Check sheet for the modelled part. Datum: model origin and axes. Units: mm. A direction names the side the tool comes from. Round coordinates to 2 decimals unless told otherwise and drop trailing zeros. Loops run counter-clockwise (first coordinate to the right, second up) from the corner with the lowest first, then second, coordinate; pieces in that order, holes last. Notation, with made-up numbers: (-1.5, 42.5) - (27.5, 42.5) arc R11 cw to (27.5, 60.5) - close; hole circle Ø7 at (29, 79.25). An arc over 180 degrees is marked (long way). Return JSON: item names as keys, results as strings.
from build123d import *

# Parameters (mm, degrees)
EXTRUDE_START            = -3.462177
EXTRUDE_1_DEPTH          = 40
EXTRUDE_START_2          = 60
EXTRUDE_2_DEPTH          = 60
CUT_EXTRUDE_1_REACH      = 163.234
CUT_EXTRUDE_1_END_RADIUS = 128.062484749
SKETCH_1_R               = 25
CUT_EXTRUDE_2_DEPTH      = 163.48076826
CUT_EXTRUDE_2_DEPTH_BACK = 163.48076826
SKETCH_5_R               = 25
SKETCH_5_R_2             = 15


with BuildPart() as part:
    # 草图2 → 凸台-拉伸1 (new body)
    with BuildSketch(Plane.XY.offset(EXTRUDE_START)):
        with BuildLine():
            Line((-80, 0), (80, 0))
            Line((80, 0), (80, 100))
            ThreePointArc((80, 100), (0, 128.062484749), (-80, 100))
            Line((-80, 100), (-80, 0))
        make_face()
    extrude(amount=-EXTRUDE_1_DEPTH)

    # 草图4 → 凸台-拉伸2 (add)
    with BuildSketch(Plane.XY.offset(-3.46217708).offset(EXTRUDE_START_2)):
        with BuildLine():
            Line((-35, 0), (-35, 123.186849948))
            ThreePointArc((-35, 123.186849948), (0, 128.062484749), (35, 123.186849948))
            Line((35, 123.186849948), (35, 0))
            Line((35, 0), (-35, 0))
        make_face()
    extrude(amount=-EXTRUDE_2_DEPTH)

    # 切除-拉伸1: up to this cylinder (the profile starts inside it)
    cut_extrude_1_end = Plane(origin=(0, 0, 6.537823), z_dir=(0, 0, 1)) * Cylinder(CUT_EXTRUDE_1_END_RADIUS, 583.592969497, mode=Mode.PRIVATE)
    # 草图1 → 切除-拉伸1 (cut, up to the surface)
    with BuildSketch(Plane(origin=(0, 0, 0), x_dir=(1, 0, 0), z_dir=(0, 1, 0)), mode=Mode.PRIVATE) as cut_extrude_1_sk1:
        with Locations(Location((0, -6.53782292, 0), (0, 0, 90))):
            Circle(SKETCH_1_R)
    cut_extrude_1_tool1 = extrude(cut_extrude_1_sk1.sketch, amount=CUT_EXTRUDE_1_REACH, mode=Mode.PRIVATE) & cut_extrude_1_end
    add(cut_extrude_1_tool1.solids().sort_by_distance((0, 0, 6.537823))[0], mode=Mode.SUBTRACT)

    # 草图5 → 切除-拉伸2 (cut, two sides: drawn at the far end of the back side and taken through both)
    with BuildSketch(Plane.XY.offset(-3.46217708).offset(-CUT_EXTRUDE_2_DEPTH_BACK)):
        with Locations((0, 70)):
            Circle(SKETCH_5_R)
        with Locations((-55, 50)):
            Circle(SKETCH_5_R_2)
        with Locations((55, 50)):
            Circle(SKETCH_5_R_2)
    extrude(amount=CUT_EXTRUDE_2_DEPTH + CUT_EXTRUDE_2_DEPTH_BACK, mode=Mode.SUBTRACT)


solid = part.part
Q1. Sectioned sample at A-A (x = -5.5). Enter the section's corners in (y, z), plus the area to 3 significant figures.
Answer key:
{"outline": "(0, -43.46) - (45.61, -43.46) - (45.61, -17.85) - (0, -17.85) - close; (0, 30.93) - (45.61, 30.93) - (45.61, 56.54) - (0, 56.54) - close; (94.39, -43.46) - (127.94, -43.46) - (127.94, -17.85) - (94.39, -17.85) - close; (94.39, 30.93) - (127.94, 30.93) - (127.94, 56.54) - (94.39, 56.54) - close", "area": "4,060 mm²"}
Q2. Scan lines: probe 1 along Z at (x, y) = (0.5, 34); probe 2 along Y at (x, z) = (0, -24); probe 3 along Z at (x, y) = (-60, 111). Record each from-to range of solid material in increasing order. Write a range as [from, to].
Answer key:
{"probe 1": "z = [-43.46, -18.46], [31.53, 56.54]", "probe 2": "y = [0, 45], [95, 128.06]", "probe 3": "z = [-43.46, -3.46]"}
Q3. Draft check along Z on faces 4 (the face through (17, 0, -15)), 5 (the face through (67, 62, -3.462)), 6 (the face through (17, 51, -43.462)), 7 (the face through (-1.099, 26.732, 31.514)). Enter one of: released by +Z, released by -Z, zero draft, split by the parting line, or undercut.
Answer key:
{"face 4": "zero draft", "face 5": "released by +Z", "face 6": "released by -Z", "face 7": "undercut"}
Q4. Sectioned sample at B-B (y = 50). Enter the section's corners in (x, z), plus the area to 3 significant figures.
Answer key:
{"outline": "(-80, -43.46) - (-70, -43.46) - (-70, -3.46) - (-80, -3.46) - close; (-40, -43.46) - (-15, -43.46) - (-15, -13.46) arc R25 cw to (-15, 26.54) - (-15, 56.54) - (-35, 56.54) - (-35, -3.46) - (-40, -3.46) - close; (15, -43.46) - (40, -43.46) - (40, -3.46) - (35, -3.46) - (35, 56.54) - (15, 56.54) - (15, 26.54) arc R25 cw to (15, -13.46) - close; (70, -43.46) - (80, -43.46) - (80, -3.46) - (70, -3.46) - close", "area": "4,640 mm²"}
Q5. Depth check by flat-ended pin: P1, Ø6, axis at x = 11, z = 30.5, coming from the +Y side; P2, Ø22.5, axis at x = -57.5, y = 61.5, coming from the +Z side; P3, Ø10, axis at x = -18.5, z = -15.5, coming from the +Y side. Enter the tip coordinate at first touch or a pass-through.
Answer key:
{"P1": "stops at y = 127.81", "P2": "stops at z = -3.46", "P3": "stops at y = 127.35"}
Q6. Sectioned sample at C-C (z = -21). Enter the section's corners in (x, y), plus the area to 3 significant figures.
Answer key:
{"outline": "(-80, 0) - (80, 0) - (80, 100) arc R128.06 ccw to (-80, 100) - close; hole circle Ø30 at (-55, 50); hole circle Ø50 at (0, 70); hole circle Ø30 at (55, 50)", "area": "15,700 mm²"}
Q7. Tool access check on faces 1 (the face through (-66.056, 60.138, -23.742)), 2 (the face through (-68, 62, -3.462)), 3 (the face through (35, 62, 27)). Record the directions out of +Z, -Z, +X, -X, +Y, -Y that give a thin tool (end or side, any length) a straight path to the whole face; none if there is none.
Answer key:
{"face 1": "+Z, -Z", "face 2": "+Z, -X, +Y, -Y", "face 3": "+Z, +X, +Y, -Y"}
Q8. Sectioned sample at D-D (y = 92). Enter the section's corners in (x, z).
Answer key:
{"outline": "(-80, -43.46) - (-11.87, -43.46) - (-11.87, -15.46) arc R25 cw to (-11.87, 28.54) - (-11.87, 56.54) - (-35, 56.54) - (-35, -3.46) - (-80, -3.46) - close; (11.87, -43.46) - (80, -43.46) - (80, -3.46) - (35, -3.46) - (35, 56.54) - (11.87, 56.54) - (11.87, 28.54) arc R25 cw to (11.87, -15.46) - close"}
